For this review, take the finished solid that the model builds, in its own axes (mm). A direction names the side the tool comes from. Coordinates: 2 decimals unless noted, no trailing zeros. Write each loop counter-clockwise with the first axis right and the second up, starting at its lowest first coordinate (ties: lowest second). Pieces come first, ordered by that corner, then holes.
```python
from build123d import *

# Parameters (mm, degrees)
F0_W   = 3
F0_H   = 10
F0_W_2 = 44
F0_H_2 = 25
F2_R   = 6
F3_W   = 3
F3_H   = 6.5
F3_W_2 = 8
F3_H_2 = 10


with BuildPart() as f1:
    # F0 (on Front) → F1 (revolve)
    with BuildSketch(Plane.XZ):
        with Locations((1.5, 11)):
            Rectangle(F0_W, F0_H)
        Polygon((-17, 6), (0, 6), (0, 16), (0, 20), (-17, 20), align=None)
        Polygon((-29, 6), (-17, 6), (-17, 20), (-17, 31), (-29, 31), align=None)
        with BuildLine():
            Line((-41, 6), (-29, 6))
            Line((-29, 6), (-29, 31))
            ThreePointArc((-29, 31), (-35, 25), (-41, 31))
            Line((-41, 31), (-41, 6))
        make_face()
        with Locations((-63, 18.5)):
            Rectangle(F0_W_2, F0_H_2)
    revolve(axis=Axis((-0.275247, 0, 0), (1, 0, 0)))

    # F2
    f2_edges = [f1.edges().sort_by_distance(p)[0] for p in [
        (-85, 0, -31),
    ]]
    fillet(f2_edges, radius=F2_R)

    # F3 (on Front) → F4 (revolve, cut)
    with BuildSketch(Plane.XZ):
        Polygon((-71.5, 16), (-83.5, 16), (-83.5, 6), (-71.5, 6), (-71.5, 12.5), align=None)
        with Locations((-70, 9.25)):
            Rectangle(F3_W, F3_H)
        Polygon((-68.5, 12.5), (-68.5, 6), (-63, 6), (-63, 16), (-63, 20.5), (-68.5, 20.5), align=None)
        with Locations((-59, 11)):
            Rectangle(F3_W_2, F3_H_2)
    revolve(axis=Axis((-38.937337, 0, 0), (1, 0, 0)), mode=Mode.SUBTRACT)


solid = f1.part
```
1) Consider section B-B (y = -14). Count the separate pieces of the cut face and the enclosed holes in it, then the cut area to 3 significant figures.
2) Clearance check with flat-ended pins moving along their axes: P1, Ø8, axis at x = -56, y = -23, coming from the +Z side; P2, Ø2, axis at x = -23, z = 13.5, coming from the -Y side; P3, Ø15, axis at y = 0, z = 0, coming from the +X side; P4, Ø5, axis at x = -42.5, z = 5.5, coming from the -Y side. State where each tip first meets the part, or that it passes through.
3) Consider section A-A (x = -60.5). Give the boundary of the cut face in (y, z), then the cut area to 3 significant figures.
4) The part is to be moulded in two halves that separate along Z. For faces 4 (the face through (-23.084, -30.736, -4.036)), 5 (the face through (-63, 11, -12)), 6 (the face through (3, 0, -7)), say which applies: pulls with the +Z half, pulls with the -Z half, needs draft (parallel to the pull), parting line crosses it, or undercut.
5) For L1, parallel to X at y = 6, z = -18.5; L2, parallel to X at y = -14, z = -6; L3, parallel to Y at x = -65, z = 0, list the stretches that pass through material, from the lowest coordinate up.
6) Tool access review of faces 1 (the face through (1.52, 15.62, -3.47)), 2 (the face through (-26, 0, -6)), 3 (the face through (-69.979, -3.755, 11.923)): name each direction out of +Z, -Z, +X, -X, +Y, -Y from which nothing blocks a thin tool from reaching the whole face with its end or side.
7) Consider section C-C (x = -21.5). Give the boundary of the cut face in (y, z), then the cut area to 3 significant figures.
Results:
1. separate pieces: 1
1. enclosed holes: 2
1. area: 3,670 mm2
2. P1: stops at z = 24.49
2. P2: stops at y = -28.37
2. P3: stops at x = 3
2. P4: stops at y = -30.85
3. outline: circle Ø62 at (0, 0); hole circle Ø32 at (0, 0)
3. area: 2,210 mm2
4. face 4: parting line crosses it
4. face 5: undercut
4. face 6: needs draft
5. L1: x = -85 to -68.5, -63 to 0
5. L2: x = -85 to -83.5, -71.5 to -68.5, -55 to 3
5. L3: y = -31 to -20.5, 20.5 to 31
6. face 1: +X
6. face 2: +X, -X
6. face 3: none
7. outline: circle Ø62 at (0, 0); hole circle Ø12 at (0, 0)
7. area: 2,910 mm2
